For this review, take the finished solid that the model builds, in its own axes (mm). A direction names the side the tool comes from. Coordinates: 2 decimals unless noted, no trailing zeros. Write each loop counter-clockwise with the first axis right and the second up, starting at its lowest first coordinate (ties: lowest second). Pieces come first, ordered by that corner, then holes.
1) We need section A-A on z = -22.5. Write out the cut boundary in (x, y), then the cut area to 3 significant figures.
2) We need section D-D on y = 27.75. Write out the cut boundary in (x, z), then the cut area to 3 significant figures.
3) For faces 1 (the face through (16, 27, -20.62)), 2 (the face through (13.64, 27, -22)), 3 (the face through (16, 27, -24.38)), 4 (the face through (18.36, 27, -22)), list the 3-axis set-ups (+Z, -Z, +X, -X, +Y, -Y) from which the entire face can be reached by the end or side of a thin tool; tool diameter is ignored.
4) We need section B-B on x = 16. Write out the cut boundary in (y, z).
5) To check wall thickness, follow line 1 along Y through (x, z) = (13.25, -24); line 2 along X through (y, z) = (26.6, -22.5); line 3 along Z through (x, y) = (15, 26.8). State the ranges of each line that lie inside material, in increasing order.
6) We need section C-C on y = 27. Write out the cut boundary in (x, z), then the cut area to 3 significant figures.
7) Insertion check: P1, Ø0.6, axis at y = 27, z = -23, coming from the +X side; P2, Ø1, axis at y = 27, z = -19.5, coming from the +X side; P3, Ø0.9, axis at x = 15.5, y = 27, coming from the -Z side. Each pin has a flat end and moves straight along its axis. Give the tip position at first contact, or say it passes through.
from build123d import *

# Parameters (mm, degrees)
PCB_SK1_R = 7.1
PCB_DEPTH = 1
MIC_SK2_W = 4.72
MIC_SK2_H = 3.76
MIC_DEPTH = 1.1


with BuildPart() as part:
    # PCB_Sk1 → PCB (new body)
    with BuildSketch(Plane(origin=(0, 28.4, 0), x_dir=(1, 0, 0), z_dir=(0, 1, 0))):
        with Locations(Location((16, 22.5, 0), (0, 0, 270))):
            Circle(PCB_SK1_R)
    extrude(amount=-PCB_DEPTH)

    # Mic_Sk2 → Mic (add)
    with BuildSketch(Plane(origin=(0, 27.4, 0), x_dir=(1, 0, 0), z_dir=(0, 1, 0))):
        with Locations((16, 22.5)):
            Rectangle(MIC_SK2_W, MIC_SK2_H)
    extrude(amount=-MIC_DEPTH)


solid = part.part
Result:
1. outline: (8.9, 27.4) - (13.64, 27.4) - (13.64, 26.3) - (18.36, 26.3) - (18.36, 27.4) - (23.1, 27.4) - (23.1, 28.4) - (8.9, 28.4) - close
1. area: 19.4 mm2
2. outline: circle Ø14.2 at (16, -22.5)
2. area: 158 mm2
3. face 1: +Z, +X, -X, -Y
3. face 2: +Z, -Z, -X, -Y
3. face 3: -Z, +X, -X, -Y
3. face 4: +Z, -Z, +X, -Y
4. outline: (26.3, -24.38) - (27.4, -24.38) - (27.4, -29.6) - (28.4, -29.6) - (28.4, -15.4) - (27.4, -15.4) - (27.4, -20.62) - (26.3, -20.62) - close
5. line 1: y = 27.4 to 28.4
5. line 2: x = 13.64 to 18.36
5. line 3: z = -24.38 to -20.62
6. outline: (13.64, -24.38) - (18.36, -24.38) - (18.36, -20.62) - (13.64, -20.62) - close
6. area: 17.7 mm2
7. P1: stops at x = 18.36
7. P2: stops at x = 22.57
7. P3: stops at z = -29.59
